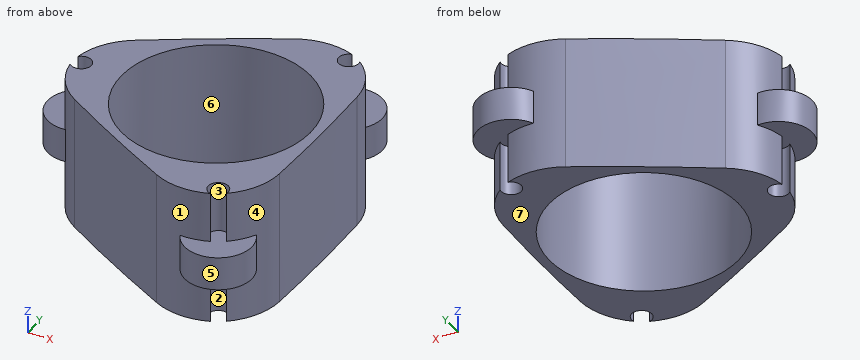
```python
from build123d import *

# Parameters (mm, degrees)
SKETCH1_R               = 14.075
BOSS_EXTRUDE1_DEPTH     = 20
FILLET2_R               = 10
CIRPATTERN2_DEPTH       = 20
CUT_EXTRUDE1_DEPTH      = 36.236736823
CUT_EXTRUDE1_DEPTH_BACK = 36.236736823
SKETCH2_R               = 1.5
SKETCH3_R               = 5
BOSS_EXTRUDE2_DEPTH     = 2.5


# Read off the part's stored shape, not the designer's step: CirPattern2
with BuildPart() as part:
    # Sketch1 → Boss-Extrude1 (new body)
    with BuildSketch(Plane.XY):
        with BuildLine():
            ThreePointArc((15.07572539, 15.156517087), (10.68875, 18.513458069), (5.588066136, 20.634219712))
            add(Edge.make_bspline(
                [(-20.663791525, 5.477702624), (-6.455161962, 14.620684981), (5.588066136, 20.634219712)],
                knots=[0, 0, 0, 1, 1, 1], degree=2))
            ThreePointArc((-20.663791525, 5.477702624), (-21.3775, 0), (-20.663791525, -5.477702624))
            add(Edge.make_bspline(
                [(5.588066136, -20.634219712), (-9.434303633, -12.900676735), (-20.663791525, -5.477702624)],
                knots=[0, 0, 0, 1, 1, 1], degree=2))
            ThreePointArc((5.588066136, -20.634219712), (10.68875, -18.513458069), (15.07572539, -15.156517087))
            add(Edge.make_bspline(
                [(15.07572539, 15.156517087), (15.889465595, -1.720008246), (15.07572539, -15.156517087)],
                knots=[0, 0, 0, 1, 1, 1], degree=2))
        make_face()
        Circle(SKETCH1_R, mode=Mode.SUBTRACT)
    extrude(amount=BOSS_EXTRUDE1_DEPTH)

    # Fillet2
    # the kernel refuses this fillet: 10 mm, written as the material it takes off along each edge
    with BuildSketch(Plane(origin=(-20.663791525, 5.477702624, 0), x_dir=(0.8442926206452175, 0.535882422480931, 0), z_dir=(0, 0, 1))) as fillet2_piece_1:
        with BuildLine():
            CenterArc((4.663228268, -9.99979423), FILLET2_R, 89.632438943, 60.311708344)
            Line((-3.992147587, -4.991354472), (-4.165255104, -4.891185677))
            ThreePointArc((-4.165255104, -4.891185677), (-2.339855889, -2.220716027), (-0.135758458, 0.146866065))
            Line((-0.135758458, 0.146866065), (-0.001245228, 0.199996123))
            ThreePointArc((-0.001245228, 0.199996123), (2.363679869, 0.207468059), (4.728662356, 0.199995885))
            Line((4.728662356, 0.199995885), (4.727379335, 0))
        make_face()
    extrude(amount=20, mode=Mode.SUBTRACT)
    with BuildSketch(Plane(origin=(-20.663791525, -5.477702624, 0), x_dir=(-0.11054249856240242, 0.9938713981253215, 0), z_dir=(0, 0, 1))) as fillet2_piece_2:
        with BuildLine():
            CenterArc((4.841664479, -9.890151004), FILLET2_R, 81.49970425, 59.972427812)
            Line((-2.981388332, -3.661198868), (-3.137849388, -3.536619825))
            ThreePointArc((-3.137849388, -3.536619825), (-1.656048683, -1.695980181), (-0.153629227, 0.128054913))
            Line((-0.153629227, 0.128054913), (-0.029562903, 0.19780302))
            ThreePointArc((-0.029562903, 0.19780302), (3.159904821, 0.434829692), (6.349372545, 0.19780302))
            Line((6.349372545, 0.19780302), (6.319809642, 0))
        make_face()
    extrude(amount=20, mode=Mode.SUBTRACT)

    # CirPattern2 outline → CirPattern2 (cut)
    with BuildSketch(Plane.XY):
        with BuildLine():
            add(Edge.make_bspline(
                [(5.588066136, 20.634219712), (3.520088132, 19.601618033), (1.388262549, 18.476743556)],
                knots=[0, 0, 0, 0.171712932, 0.171712932, 0.171712932], degree=2))
            ThreePointArc((1.388262549, 18.476743556), (6.013402902, 19.632371585), (10.648001522, 18.515279353))
            ThreePointArc((10.648001522, 18.515279353), (13.959170177, 15.045625026), (15.27399868, 10.43329752))
            add(Edge.make_bspline(
                [(15.27399868, 10.43329752), (15.191267831, 12.760230261), (15.07572539, 15.156517087)],
                knots=[0.858010652, 0.858010652, 0.858010652, 1, 1, 1], degree=2))
            ThreePointArc((15.07572539, 15.156517087), (10.68875, 18.513458069), (5.588066136, 20.634219712))
        make_face()
        with BuildLine():
            add(Edge.make_bspline(
                [(15.07572539, -15.156517087), (15.215455106, -12.849294762), (15.307198024, -10.440642412)],
                knots=[0, 0, 0, 0.171712932, 0.171712932, 0.171712932], degree=2))
            ThreePointArc((15.307198024, -10.440642412), (13.995431078, -15.023945468), (10.710701517, -18.479079494))
            ThreePointArc((10.710701517, -18.479079494), (6.0503084, -19.611808503), (1.398501358, -18.444319635))
            add(Edge.make_bspline(
                [(1.398501358, -18.444319635), (3.455049649, -19.536138988), (5.588066136, -20.634219712)],
                knots=[0.858010652, 0.858010652, 0.858010652, 1, 1, 1], degree=2))
            ThreePointArc((5.588066136, -20.634219712), (10.68875, -18.513458069), (15.07572539, -15.156517087))
        make_face()
    extrude(amount=CIRPATTERN2_DEPTH, mode=Mode.SUBTRACT)

    # Sketch2 → Cut-Extrude1 (cut, two sides: drawn at the far end of the back side and taken through both)
    with BuildSketch(Plane.XY.offset(20).offset(-CUT_EXTRUDE1_DEPTH_BACK)):
        with Locations((10.084522584, -17.466905485)):
            Circle(SKETCH2_R)
        with Locations((10.084522584, 17.466905485)):
            Circle(SKETCH2_R)
        with Locations((-20.169045167, 0)):
            Circle(SKETCH2_R)
    extrude(amount=CUT_EXTRUDE1_DEPTH + CUT_EXTRUDE1_DEPTH_BACK, mode=Mode.SUBTRACT)

    # Sketch3 → Boss-Extrude2 (add, symmetric)
    with BuildSketch(Plane.XY.offset(10)):
        with Locations((-20.169045167, 0)):
            Circle(SKETCH3_R)
        with Locations((10.084522584, 17.466905485)):
            Circle(SKETCH3_R)
        with Locations((10.084522584, -17.466905485)):
            Circle(SKETCH3_R)
    extrude(amount=BOSS_EXTRUDE2_DEPTH, both=True)


solid = part.part
```
Source: CAD feature listing. Evaluate the final solid. Frame: model axes, mm. Face numbers are marked on the shaded views. A direction names the side the tool comes from. Round coordinates to 2 decimals unless told otherwise and drop trailing zeros. Loops run counter-clockwise (first coordinate to the right, second up) from the corner with the lowest first, then second, coordinate; pieces in that order, holes last. Notation, with made-up numbers: M 67.25,-21.75 L 91.25,-21.75 A33 ccw 91.25,14.25 Z; hole C 43,41.25 d4. An arc over 180 degrees is marked long. Put each result on its own line as item: value.
(1) Ray query, line 1 (Y direction, x = -1, z = 6); line 2 (Y direction, x = 4, z = 16.75); line 3 (X direction, y = 12.5, z = 7.75). Return the intervals inside material, ascending. Write a range as [from, to].
Solutions:
line 1: [-17.16, -14.04], [14.04, 17.2]
line 2: [-19.39, -13.49], [13.49, 19.42]
line 3: [-9.29, -6.47], [6.47, 14.98]
(2) Section A-A, the plane x = -22. Return loops of the section in (y, z), and give its area (3 significant figures).
Solutions:
outline: M -4.65,7.5 L 4.65,7.5 L 4.65,12.5 L -4.65,12.5 Z
area: 46.5 mm²
(3) Pull-direction query (X, two-part tool) for the marked faces 4, 5, 6 and 7; classes: released by +X, released by -X, zero draft, split by the parting line, or undercut.
Solutions:
face 4: released by +X
face 5: split by the parting line
face 6: undercut
face 7: zero draft
(4) Access query for the marked faces 1, 2 and 3. Directions: +Z, -Z, +X, -X, +Y, -Y. A direction counts if a zero-diameter tool reaches every point of the face in a straight line with its end or side. Return the directions, or none.
Solutions:
face 1: -Y
face 2: -Z
face 3: +Z
(5) First-contact query: pin 1 (2.5 mm diameter, centred on x = 10.08, y = -17.47, fed in from +Z); pin 2 (6 mm diameter, centred on x = -9.5, z = 6, fed in from +Y); pin 3 (6 mm diameter, centred on x = 10, y = 1, fed in from +Z); pin 4 (1.5 mm diameter, centred on x = 4.5, z = 17.5, fed in from +Y). Flat tips, straight axial feed; report the tip coordinate or a pass-through.
Solutions:
pin 1: z = 12.5
pin 2: y = 14.12
pin 3: through
pin 4: y = 19.6
